Geometry: final body of the model. Coordinates: model frame, mm. A direction names the side the tool comes from. Give positions to 0.01 mm unless a question says otherwise; leave off trailing zeros. Write each loop counter-clockwise with the first axis right and the second up, starting at its lowest first coordinate (ties: lowest second). Pieces come first, ordered by that corner, then holes. Notation, with made-up numbers: (54, -33.5) -> (84, -33.5) arc R24 cw to (84, -19.5) -> close; hole circle Ø7 at (41.5, 82). An arc over 180 degrees is marked (long way). Answer as a JSON object with one key per item and string values.
from build123d import *

# Parameters (mm, degrees)
F0_W      = 25
F0_H      = 35
F1_DEPTH  = 4
F2_W      = 25
F2_H      = 25
F2_H_2    = 5
F3_DEPTH  = 15
F4_R      = 5
F5_W      = 15
F5_H      = 12.5
F6_DEPTH  = 11
F9_D      = 3.3
F11_DEPTH = 5.5
F7_W      = 20
F7_H      = 1.6
F12_DEPTH = 25
F14_D     = 10.0838


# Not quite as in the source:
# - a feature names something its author has since deleted; it is built from what else it names


with BuildPart() as f1:
    # F0 (on Top) → F1 (new body)
    with BuildSketch(Plane.XY):
        Rectangle(F0_W, F0_H)
    extrude(amount=F1_DEPTH)

    # F2 (on face) → F3 (join)
    with BuildSketch(Plane.XY.offset(4)):
        Rectangle(F2_W, F2_H)
        with Locations((0, -15)):
            Rectangle(F2_W, F2_H_2)
    extrude(amount=F3_DEPTH)

    # F4
    f4_edges = [f1.edges().sort_by_distance(p)[0] for p in [
        (-12.5, -2.5, 19),
        (12.5, -2.5, 19),
    ]]
    fillet(f4_edges, radius=F4_R)

    # F5 (on face) → F6 (cut)
    with BuildSketch(Plane.XY.offset(19)):
        Polygon((-16.3788758218, 17.6315885037), (-16.3788758218, 0), (-7.5, 0), (-7.5, 12.5), (7.5, 12.5), (7.5, 0), (18.287928775, 0), (18.287928775, 17.6315885037), align=None)
        with Locations((0, 6.25)):
            Rectangle(F5_W, F5_H)
    extrude(amount=-F6_DEPTH, mode=Mode.SUBTRACT)

    # F9 (through all)
    with Locations(Plane.XY.offset(8)):
        with Locations((6.6282246262, 6.25), (-6.6282246262, 6.25)):
            Hole(F9_D / 2)

    # F10 (on face) → F11 (cut)
    with BuildSketch(Plane.XY):
        Polygon((-5.0405113859, 3.5), (-3.4527981456, 6.25), (-5.0405113859, 9), (-8.2159378665, 9), (-9.8036511067, 6.25), (-8.2159378665, 3.5), align=None)
        Polygon((5.0405113859, 9), (3.4527981456, 6.25), (5.0405113859, 3.5), (8.2159378665, 3.5), (9.8036511067, 6.25), (8.2159378665, 9), align=None)
    extrude(amount=F11_DEPTH, mode=Mode.SUBTRACT)

    # F7 (on face) → F12 (cut)
    with BuildSketch(Plane.YZ.offset(12.5)):
        with Locations((8.9099199928, 3.2)):
            Rectangle(F7_W, F7_H)
    extrude(amount=-F12_DEPTH, mode=Mode.SUBTRACT)

    # F14 (through all)
    with Locations(Plane.XY.offset(19)):
        with Locations((0, -8.75)):
            Hole(F14_D / 2)


solid = f1.part
Q1. Material intervals for L1, parallel to Y at x = 0, z = 11.25; L2, parallel to Z at x = 9.5, y = 5.5; L3, parallel to Y at x = 8, z = 1.75, sorted ascending. Write a range as from..to.
Values:
{"L1": "-17.5..-13.79, -3.71..0", "L2": "0..2.4, 4..8", "L3": "-17.5..3.5, 9..17.5"}
Q2. Cut plane B-B (z = 11.75). Return the cut outline in (x, y).
Values:
{"outline": "(-12.5, -17.5) -> (12.5, -17.5) -> (12.5, 0) -> (-12.5, 0) -> close; hole circle Ø10.08 at (0, -8.75)"}
Q3. Cut plane A-A (y = -8.75). Return the cut outline in (x, z), and give its area (3 significant figures).
Values:
{"outline": "(-12.5, 0) -> (-5.04, 0) -> (-5.04, 19) -> (-7.5, 19) arc R5 ccw to (-12.5, 14) -> close; (5.04, 0) -> (12.5, 0) -> (12.5, 14) arc R5 ccw to (7.5, 19) -> (5.04, 19) -> close", "area": "273 mm²"}
Q4. Cut plane C-C (x = 0). Return the cut outline in (y, z).
Values:
{"outline": "(-17.5, 0) -> (-13.79, 0) -> (-13.79, 19) -> (-17.5, 19) -> close; (-3.71, 0) -> (17.5, 0) -> (17.5, 2.4) -> (-1.09, 2.4) -> (-1.09, 4) -> (12.5, 4) -> (12.5, 8) -> (0, 8) -> (0, 19) -> (-3.71, 19) -> close"}
Q5. Mould query, pull axis X, two halves, no side actions, for faces 1 (the cylindrical face through (11.07, -8.63, 17.5)), 2 (the flat face through (0, 6, 4)), 3 (the flat face through (9, 4.86, 4.74)). Classes: pulls with the +X half, pulls with the -X half, needs draft (parallel to the pull), parting line crosses it, or undercut.
Values:
{"face 1": "pulls with the +X half", "face 2": "needs draft", "face 3": "undercut"}
Q6. Cut plane D-D (z = 5). Return the cut outline in (x, y), and give its area (3 significant figures).
Values:
{"outline": "(-12.5, -17.5) -> (12.5, -17.5) -> (12.5, 12.5) -> (-12.5, 12.5) -> close; hole (-9.8, 6.25) -> (-8.22, 3.5) -> (-5.04, 3.5) -> (-3.45, 6.25) -> (-5.04, 9) -> (-8.22, 9) -> close; hole circle Ø10.08 at (0, -8.75); hole (3.45, 6.25) -> (5.04, 3.5) -> (8.22, 3.5) -> (9.8, 6.25) -> (8.22, 9) -> (5.04, 9) -> close", "area": "618 mm²"}
Q7. First-contact query: P1, Ø1.2, axis at x = -3.5, z = 5.5, coming from the +Y side; P2, Ø3.5, axis at x = 0.5, z = 14.5, coming from the +Y side; P3, Ø4, axis at x = -6.63, y = 6.25, coming from the -Z side. Flat tips, straight axial feed; report the tip coordinate or a pass-through.
Values:
{"P1": "y = 12.5", "P2": "y = 0", "P3": "z = 5.5"}
Q8. Set-up query: faces 4 (the flat face through (-9, 7.64, 1.18)), 5 (the flat face through (-3.4, -4.7, 19)). Return all of +Z, -Z, +X, -X, +Y, -Y with unobstructed straight access to the full face (end or side cutting, diameter ignored); none if empty.
Values:
{"face 4": "-Z", "face 5": "+Z, +X, -X, +Y, -Y"}
